Part model, mm, in its own coordinate system. A direction names the side the tool comes from. Give positions to 0.01 mm unless a question says otherwise; leave off trailing zeros. Order: outer loops, then holes, each group sorted by start corner. A loop starts at its lowest first (then second) coordinate and runs counter-clockwise, first axis right, second up. Notation, with made-up numbers: M 64.5,-39 L 99.5,-39 A11 cw 99.5,-21 Z; hole C -26,30.5 d7. An arc over 180 degrees is marked long. One line per question, with ' | ' between items.
Autodesk Inventor part; units mm, degrees
ref_plane "YZ Plane" through (0, 0, 0) normal (1, 0, 0) x (0, 1, 0)
ref_plane "XZ Plane" through (0, 0, 0) normal (0, 1, 0) x (-1, 0, 0)
ref_plane "XY Plane" through (0, 0, 0) normal (0, 0, 1) x (1, 0, 0)
sketch "Base" plane through (0, 0, 0) normal (0, 0, 1) x (1, 0, 0)
  circle A0 centre (0, 0) radius 10.25
  dimension "d0" = 20.5
extrude "BaseFeature" add sketch "Base" along normal mid plane 16
sketch "Ridges" plane through (0, 0, 0) normal (0, 0, 1) x (1, 0, 0)
  circle A0 centre (0, 0) radius 10.25
  circle A1 centre (0, 0) radius 7.5
  dimension "d3" = 15
extrude "RidgesFeature" cut sketch "Ridges" along normal mid plane 12.25
sketch "Countersink" plane through (0, 0, 8) normal (0, 0, 1) x (1, 0, 0)
  circle A0 centre (0, 0) radius 6.5
  dimension "d6" = 13
extrude "CountersinkFeature" cut sketch "Countersink" against normal blind 3
mirror "CountersinkMirrorFeature" about plane through (0, 0, 0) normal (0, 0, 1) of "CountersinkFeature"
sketch "MountHole" plane through (0, 0, 5) normal (0, 0, 1) x (1, 0, 0)
  point P0 (0, 0)
hole "MountHoleFeature" at (0, 0, 5) direction (0, 0, -1) diameter 6 end through all
properties part number "LegChainTensionerBlock"
1. Mould opens along Z. For faces 1 (the flat face through (3, -1, 5)), 2 (the flat face through (0, -7, -8)), 3 (the flat face through (1, -8, -6.125)) say: released by +Z, released by -Z, zero draft, split by the parting line, or undercut.
Worked out:
face 1: released by +Z | face 2: released by -Z | face 3: undercut
2. Drop flat-ended pins along their axis: pin 1 (9.5 mm diameter, centred on x = 0, y = 0, fed in from +Z); pin 2 (4 mm diameter, centred on y = 1, z = -3, fed in from +X); pin 3 (1.5 mm diameter, centred on x = -6.5, z = -3, fed in from +Y). Give the stop position or say it passes through.
Worked out:
pin 1: stops at z = 5 | pin 2: stops at x = 7.5 | pin 3: stops at y = 4.82
3. Tool access for faces 4 (the flat face through (1, -8, 6.125)), 5 (the flat face through (0, -7, 8)), 6 (the cylindrical face through (-5.158, -3.955, 6.521)), 7 (the cylindrical face through (-5.158, 3.955, -6.521)): list every direction of +Z, -Z, +X, -X, +Y, -Y with a clear straight run to the whole face (end or side of a thin tool).
Worked out:
face 4: none | face 5: +Z, +X, -X, +Y, -Y | face 6: +Z | face 7: -Z
4. Slice it at A-A on x = 0. Give the cut face in (y, z) (3 decimals), then the cut area to 3 significant figures.
Worked out:
outline: M -10.25,-8 L -6.5,-8 L -6.5,-5 L -3,-5 L -3,5 L -6.5,5 L -6.5,8 L -10.25,8 L -10.25,6.125 L -7.5,6.125 L -7.5,-6.125 L -10.25,-6.125 Z; M 3,-5 L 6.5,-5 L 6.5,-8 L 10.25,-8 L 10.25,-6.125 L 7.5,-6.125 L 7.5,6.125 L 10.25,6.125 L 10.25,8 L 6.5,8 L 6.5,5 L 3,5 Z | area: 123 mm2
5. Slice it at C-C on z = 3. Give the cut face in (x, y), then the cut area to 3 significant figures.
Worked out:
outline: C 0,0 d15; hole C 0,0 d6 | area: 148 mm2
6. Probe L1, parallel to Y at x = 0, z = 7.35; L2, parallel to Z at x = 5.25, y = -7 (3 decimals); L3, parallel to Z at x = 3, y = -1. List the from-to ranges inside material, lowest first. Write a range as from..to.
Worked out:
L1: y = -10.25..-6.5, 6.5..10.25 | L2: z = -8..-6.125, 6.125..8 | L3: z = -5..5
7. Slice it at D-D on y = -5.5. Give the cut face in (x, z) (3 decimals).
Worked out:
outline: M -8.649,-8 L -3.464,-8 L -3.464,-5 L 3.464,-5 L 3.464,-8 L 8.649,-8 L 8.649,-6.125 L 5.099,-6.125 L 5.099,6.125 L 8.649,6.125 L 8.649,8 L 3.464,8 L 3.464,5 L -3.464,5 L -3.464,8 L -8.649,8 L -8.649,6.125 L -5.099,6.125 L -5.099,-6.125 L -8.649,-6.125 Z
